Autodesk Inventor part; units mm, degrees
ref_plane "YZ Plane" through (0, 0, 0) normal (1, 0, 0) x (0, 1, 0)
ref_plane "XZ Plane" through (0, 0, 0) normal (0, 1, 0) x (-1, 0, 0)
ref_plane "XY Plane" through (0, 0, 0) normal (0, 0, 1) x (1, 0, 0)
sketch "Sketch1" plane through (0, 0, 0) normal (0, 0, 1) x (1, 0, 0)
  circle A0 centre (0, 0) radius 12.5
  dimension "d0" = 25
extrude "Extrusion1" add sketch "Sketch1" along normal blind 25
chamfer "Chamfer2" distance 2 angle 45 1 edges at (-12.5, 0, 0)
sketch "Sketch2" plane through (0, 0, 0) normal (1, 0, 0) x (0, 1, 0)
  line L0 (0, 0) -> (1, 0)
  line L1 (1, 0) -> (1, 4)
  line L2 (1, 4) -> (0, 4)
  line L3 (0, 4) -> (0, 0)
  line L4 (12.5, 25) -> (-12.5, 25)
  line L5 (0, 4) -> (2.575, 4)
  line L6 (2.575, 4) -> (2.575, 25)
  line L7 (2.575, 25) -> (0, 25)
  line L8 (0, 25) -> (0, 4)
  line L9 (2.575, 4) -> (1, 2.685)
  line L10 (1, 2.685) -> (0, 1.85) construction
  dimension "d9" = 1
  dimension "d10" = 2.575
  dimension "d11" = 4
  dimension "d42" = 2.15
revolve "Revolution1" cut sketch "Sketch2" angle 360 about axis through (0, 0, 25) along (0, 0, -1)
chamfer "Chamfer3" distance 1 angle 45 2 edges at (0, -1, 0) (0, -2.575, 25)
sketch "Sketch3" plane through (0, 0, 25) normal (0, 0, 1) x (1, 0, 0)
  circle A0 centre (0, 0) radius 9
  line L0 (0, 0) -> (26.029, 0) construction
  circle A1 centre (0, 0) radius 12.5 construction
  circle A2 centre (12.5, 0) radius 2.5
  circle A3 centre (0, 12.5) radius 2.5
  circle A4 centre (-12.5, 0) radius 2.5
  circle A5 centre (0, -12.5) radius 2.5
  circle A6 centre (0, 0) radius 12.5
  point P0 (-2.4875, 12.25)
  point P1 (-12.25, 2.4875)
  point P2 (-12.25, -2.4875)
  point P3 (-2.4875, -12.25)
  point P4 (2.4875, -12.25)
  point P5 (12.25, -2.4875)
  point P6 (12.25, 2.4875)
  point P7 (2.4875, 12.25)
  dimension "d16" = 5
  dimension "d19" = 360
  dimension "d21" = 25
  dimension "d22" = 18
extrude "Extrusion2" cut sketch "Sketch3" against normal through all contours A2 A6 | A6 A2 | A6 A3 | A3 A6 | A6 A5 | A5 A6 | A6 A4 | A4 A6
extrude "Extrusion3" cut sketch "Sketch3" against normal blind 5 contours A2 A6 A5 A4 A3
chamfer "Chamfer4" distance 1 angle 45 5 edges at (-9, 0, 25) (-8.8388, -8.8388, 20) (8.8388, -8.8388, 20) (8.8388, 8.8388, 20) (-8.8388, 8.8388, 20)
sketch "Sketch4" plane through (0, 0, 20) normal (0, 0, 1) x (1, 0, 0)
  line L0 (0, 0) -> (-18.6595, 0) construction
  line L1 (0, 0) -> (0, 25.4609) construction
  circle A0 centre (0, 0) radius 2.575 construction
  line L2 (0, 0) -> (-16.5294, 16.5294) construction
  circle A1 centre (-7.4246, 7.4246) radius 0.75
  circle A2 centre (0, 0) radius 3.575 construction
  circle A3 centre (0, 0) radius 10.5 construction
  circle A4 centre (-7.4246, -7.4246) radius 0.75
  circle A5 centre (7.4246, -7.4246) radius 0.75
  circle A6 centre (7.4246, 7.4246) radius 0.75
  point P0 (0, 0)
  dimension "d31" = 21
  dimension "d30" = 45
  dimension "d32" = 1.5
  dimension "d35" = 360
extrude "Extrusion4" add sketch "Sketch4" along normal blind 1.5
chamfer "Chamfer5" distance 0.35 angle 45 4 edges at (6.6746, 7.4246, 21.5) (-8.1746, 7.4246, 21.5) (-8.1746, -7.4246, 21.5) (6.6746, -7.4246, 21.5)
properties part number "centrifugetool_5mm_base_v2"
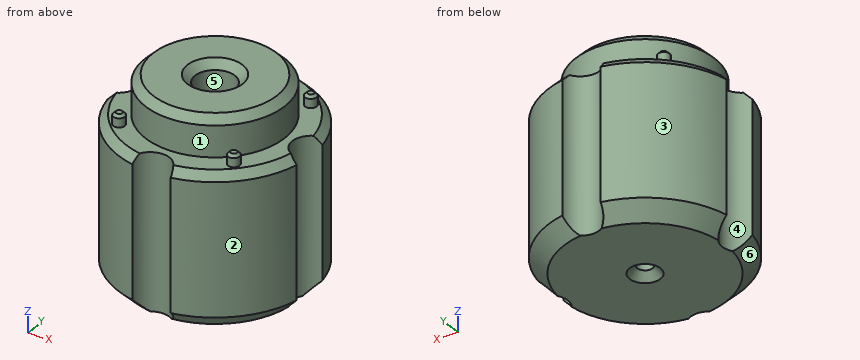
Here's how the part is built. I have some questions about the finished solid (model axes, mm). Face numbers are marked on the shaded views. A direction names the side the tool comes from. Round coordinates to 2 decimals unless told otherwise and drop trailing zeros. Loops run counter-clockwise (first coordinate to the right, second up) from the corner with the lowest first, then second, coordinate; pieces in that order, holes last. Notation, with made-up numbers: (53, 68) -> (73, 68) arc R5 ccw to (73, 74) -> close; hole circle Ø9 at (53.25, 19.5). An arc over 180 degrees is marked (long way). Answer as CSV lines item,"result".
1. Thinking about a two-plate mould opening in Y: for the marked faces 3, 4, 5 and 6, which applies, released by +Y, released by -Y, zero draft, split by the parting line, or undercut?
Final values:
face 3,"released by +Y"
face 4,"undercut"
face 5,"undercut"
face 6,"released by -Y"
2. If we section it at A-A on x = 0: Please give me the cut outline in (y, z) (3 decimals).
Final values:
outline,"(-10, 0) -> (-2, 0) -> (-1, 1) -> (-1, 2.685) -> (-2.575, 4) -> (-2.575, 24) -> (-3.575, 25) -> (-8, 25) -> (-9, 24) -> (-9, 20) -> (-10, 20) -> close; (1, 1) -> (2, 0) -> (10, 0) -> (10, 20) -> (9, 20) -> (9, 24) -> (8, 25) -> (3.575, 25) -> (2.575, 24) -> (2.575, 4) -> (1, 2.685) -> close"
3. Which directions (+Z, -Z, +X, -X, +Y, -Y) give clear straight access to the entire face, cutting with the end or side of a thin tool? Please do the marked faces 1 and 2.
Final values:
face 1,"+Z"
face 2,"+Z, -Z, +X, -Y"
4. For pin 1 (0.6 mm diameter, centred on x = -7.5, y = -7.5, fed in from +Z); pin 2 (6 mm diameter, centred on x = -2.5, y = -0.5, fed in from -Z); pin 3 (5 mm diameter, centred on y = -7.5, z = 11, fed in from -X); pin 4 (5 mm diameter, centred on x = -7, z = 11.5, fed in from -Y), each with a flat end and sliding along its axis, tell me the tip position at first contact or that it passes through.
Final values:
pin 1,"stops at z = 21.5"
pin 2,"stops at z = 0"
pin 3,"stops at x = -11.46"
pin 4,"stops at y = -11.66"
5. If we section it at C-C on z = 8.5: Please give me the cut outline in (x, y) (3 decimals).
Final values:
outline,"(-12.25, -2.487) arc R12.5 ccw to (-2.487, -12.25) arc R2.5 cw to (2.487, -12.25) arc R12.5 ccw to (12.25, -2.487) arc R2.5 cw to (12.25, 2.487) arc R12.5 ccw to (2.487, 12.25) arc R2.5 cw to (-2.487, 12.25) arc R12.5 ccw to (-12.25, 2.487) arc R2.5 cw to start; hole circle Ø5.15 at (0, 0)"
6. If I drill on L1, parallel to X at y = 0, z = 1.95; L2, parallel to X at y = 0, z = 15.25 (3 decimals); L3, parallel to Z at x = 9.5, y = 1.25, over which ranges is the centre line in solid material (lowest first)?
Final values:
L1,"x = -10 to -1, 1 to 10"
L2,"x = -10 to -2.575, 2.575 to 10"
L3,"z = 0 to 20"
